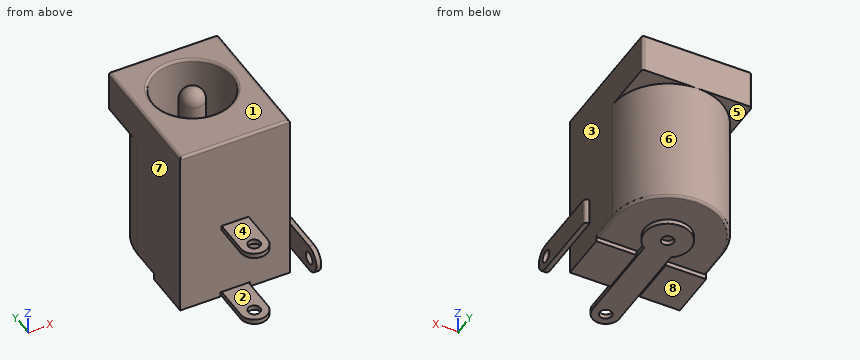
```python
from build123d import *

# Parameters (mm, degrees)
SKETCH1_W           = 9
SKETCH1_H           = 11
BOSS_EXTRUDE1_DEPTH = 3.3
BOSS_EXTRUDE2_DEPTH = 11
SKETCH3_R           = 3.25
CUT_EXTRUDE1_DEPTH  = 11
SKETCH4_R           = 1
BOSS_EXTRUDE3_DEPTH = 11
FILLET1_R           = 1
FILLET2_R           = 0.2
CUT_EXTRUDE2_DEPTH  = 0.4
SKETCH6_R           = 0.5
BOSS_EXTRUDE4_DEPTH = 0.4
SKETCH7_R           = 1.9
SKETCH7_R_2         = 0.5
BOSS_EXTRUDE5_DEPTH = 0.4
SKETCH8_R           = 0.5
BOSS_EXTRUDE6_DEPTH = 0.4
SKETCH9_R           = 0.5
BOSS_EXTRUDE7_DEPTH = 0.4
SKETCH10_W          = 2.8
SKETCH10_H          = 1
BOSS_EXTRUDE8_DEPTH = 6.4
FILLET3_R           = 0.3
FILLET4_R           = 0.2


with BuildPart() as part:
    # Sketch1 → Boss-Extrude1 (new body)
    with BuildSketch(Plane.XY):
        Rectangle(SKETCH1_W, SKETCH1_H)
    extrude(amount=-BOSS_EXTRUDE1_DEPTH)

    # Sketch2 → Boss-Extrude2 (add)
    with BuildSketch(Plane(origin=(0, 0, -3.3), x_dir=(-1, 0, 0), z_dir=(0, 0, -1))):
        with BuildLine():
            Line((-4.5, -5.5), (4.5, -5.5))
            Line((4.5, -5.5), (4.5, 1))
            ThreePointArc((4.5, 1), (0, 5.5), (-4.5, 1))
            Line((-4.5, 1), (-4.5, -5.5))
        make_face()
    extrude(amount=BOSS_EXTRUDE2_DEPTH)

    # Sketch3 → Cut-Extrude1 (cut)
    with BuildSketch(Plane.XY):
        with Locations((0, 1)):
            Circle(SKETCH3_R)
    extrude(amount=-CUT_EXTRUDE1_DEPTH, mode=Mode.SUBTRACT)

    # Sketch4 → Boss-Extrude3 (add)
    with BuildSketch(Plane.XY.offset(-11)):
        with Locations((0, 1)):
            Circle(SKETCH4_R)
    extrude(amount=BOSS_EXTRUDE3_DEPTH)

    # Fillet1
    fillet1_edges = [part.edges().sort_by_distance(p)[0] for p in [
        (-1, 1, 0),
    ]]
    fillet(fillet1_edges, radius=FILLET1_R)

    # Fillet2
    fillet2_edges = [part.edges().sort_by_distance(p)[0] for p in [
        (-3.25, 1, 0),
        (0, -5.5, 0),
        (-4.5, 0, 0),
        (0, 5.5, 0),
        (4.5, 0, 0),
        (-4.5, 5.5, -1.65),
        (4.5, 5.5, -1.65),
    ]]
    fillet(fillet2_edges, radius=FILLET2_R)

    # Sketch5 → Cut-Extrude2 (cut)
    with BuildSketch(Plane(origin=(0, 0, -14.3), x_dir=(-1, 0, 0), z_dir=(0, 0, -1))):
        Polygon((4.5, -1.5), (1.2, -1.5), (1.2, -5.5), (-1.2, -5.5), (-1.2, -1.5), (-4.5, -1.5), (-4.5, 5.5), (4.5, 5.5), align=None)
    extrude(amount=-CUT_EXTRUDE2_DEPTH, mode=Mode.SUBTRACT)

    # Sketch6 → Boss-Extrude4 (add)
    with BuildSketch(Plane(origin=(0, 0, -13.9), x_dir=(-1, 0, 0), z_dir=(0, 0, -1))):
        with BuildLine():
            Line((-1.1, -8.4), (-1.1, 1))
            ThreePointArc((-1.1, 1), (0, 2.1), (1.1, 1))
            Line((1.1, 1), (1.1, -8.4))
            ThreePointArc((1.1, -8.4), (0, -9.5), (-1.1, -8.4))
        make_face()
        with Locations((0, -8.4)):
            Circle(SKETCH6_R, mode=Mode.SUBTRACT)
        with Locations((0, 1)):
            Circle(SKETCH6_R, mode=Mode.SUBTRACT)
    extrude(amount=BOSS_EXTRUDE4_DEPTH)

    # Sketch7 → Boss-Extrude5 (add)
    with BuildSketch(Plane(origin=(0, 0, -14.3), x_dir=(-1, 0, 0), z_dir=(0, 0, -1))):
        with Locations((0, 1)):
            Circle(SKETCH7_R)
        with Locations((0, 1)):
            Circle(SKETCH7_R_2, mode=Mode.SUBTRACT)
    extrude(amount=-BOSS_EXTRUDE5_DEPTH)

    # Sketch8 → Boss-Extrude6 (add)
    with BuildSketch(Plane(origin=(0, 0, -8.1), x_dir=(-1, 0, 0), z_dir=(0, 0, -1))):
        with BuildLine():
            Line((-1.1, -5.145239298), (-1.1, -8.4))
            ThreePointArc((-1.1, -8.4), (0, -9.5), (1.1, -8.4))
            Line((1.1, -8.4), (1.1, -5.145239298))
            Line((1.1, -5.145239298), (-1.1, -5.145239298))
        make_face()
        with Locations((0, -8.4)):
            Circle(SKETCH8_R, mode=Mode.SUBTRACT)
    extrude(amount=-BOSS_EXTRUDE6_DEPTH)

    # Sketch9 → Boss-Extrude7 (add)
    with BuildSketch(Plane(origin=(4.5, 0, 0), x_dir=(0, 0, -1), z_dir=(1, 0, 0))):
        with BuildLine():
            Line((9.7, -2.5), (9.7, -8.4))
            ThreePointArc((9.7, -8.4), (10.8, -9.5), (11.9, -8.4))
            Line((11.9, -8.4), (11.9, -2.5))
            Line((11.9, -2.5), (9.7, -2.5))
        make_face()
        with Locations((10.8, -8.4)):
            Circle(SKETCH9_R, mode=Mode.SUBTRACT)
    extrude(amount=BOSS_EXTRUDE7_DEPTH)

    # Sketch10 → Boss-Extrude8 (add)
    with BuildSketch(Plane.XY.offset(-11)):
        with Locations((0, -2.25)):
            Rectangle(SKETCH10_W, SKETCH10_H)
    extrude(amount=BOSS_EXTRUDE8_DEPTH)

    # Fillet3
    fillet3_edges = [part.edges().sort_by_distance(p)[0] for p in [
        (4.9, -2.5, -10.8),
        (0, -1.75, -4.6),
    ]]
    fillet(fillet3_edges, radius=FILLET3_R)

    # Fillet4
    fillet4_edges = [part.edges().sort_by_distance(p)[0] for p in [
        (0, 5.5, -13.9),
        (4.5, -0.25, -13.9),
        (-4.5, -0.25, -13.9),
    ]]
    fillet(fillet4_edges, radius=FILLET4_R)


solid = part.part
```
Read the model definition and answer for the solid it produces. Units are mm, in the model's axes. Face numbers are marked on the shaded views. A direction names the side the tool comes from. Round coordinates to 2 decimals unless told otherwise and drop trailing zeros. Write each loop counter-clockwise with the first axis right and the second up, starting at its lowest first coordinate (ties: lowest second). Pieces come first, ordered by that corner, then holes. Notation, with made-up numbers: (4, 81) -> (13, 81) arc R24 ccw to (13, 117) -> close; hole circle Ø7 at (58, 14). An arc over 180 degrees is marked (long way). Answer in a Markdown table with one row per item. Add a question column.
1) Find section C-C, the plane z = -8.75. Determine the outline of the cut face in (x, y).
2) Given P1, Ø2.5, axis at x = 0, y = -8, coming from the +Z side; P2, Ø4, axis at x = -0.5, z = -8, coming from the -Y side; P3, Ø1.5, axis at y = -3, z = -6, coming from the +X side; P4, Ø0.7, axis at x = 3, z = -14, coming from the +Y side, each flat-ended and moving along its own axis, determine where each tip first touches the part or whether it passes through.
3) Determine the mould class of the marked faces 1, 2 and 3 for opening direction Z: pulls with the +Z half, pulls with the -Z half, needs draft (parallel to the pull), parting line crosses it, or undercut.
4) Find section A-A, the plane z = -1.75. Determine the outline of the cut face in (x, y).
5) Find section D-D, the plane z = -3.5. Determine the outline of the cut face in (x, y), and give its area (3 significant figures).
6) Which of the six approach directions +Z, -Z, +X, -X, +Y, -Y give full straight-line access (tool end or side, diameter ignored) to the marked faces 4, 5, 6, 7 and 8?
7) Consider line 1 (Y direction, x = 0, z = -14.05); line 2 (Y direction, x = 0, z = -7.9); line 3 (Y direction, x = 0, z = -5.75). Determine where each line is inside the solid, lowest interval first.
8) Find section B-B, the plane z = -10.8. Determine the outline of the cut face in (x, y).
Findings below:
| question | item | result |
|---|---|---|
| 1 | outline | (-4.5, -5.5) -> (4.5, -5.5) -> (4.5, 1) arc R4.5 ccw to (-4.5, 1) -> close; circle Ø2 at (0, 1); hole (-1.4, -1.93) -> (-1.4, -1.75) -> (1.4, -1.75) -> (1.4, -1.93) arc R3.25 ccw (long way) to start |
| 2 | P1 | z = -7.7 |
| 2 | P2 | y = -9.5 |
| 2 | P3 | x = 4.5 |
| 2 | P4 | y = 4.56 |
| 3 | face 1 | pulls with the +Z half |
| 3 | face 2 | undercut |
| 3 | face 3 | needs draft |
| 4 | outline | (-4.5, -5.5) -> (4.5, -5.5) -> (4.5, 5.3) arc R0.2 ccw to (4.3, 5.5) -> (-4.3, 5.5) arc R0.2 ccw to (-4.5, 5.3) -> close; circle Ø2 at (0, 1); hole circle Ø6.5 at (0, 1) |
| 5 | outline | (-4.5, -5.5) -> (4.5, -5.5) -> (4.5, 1) arc R4.5 ccw to (-4.5, 1) -> close; circle Ø2 at (0, 1); hole circle Ø6.5 at (0, 1) |
| 5 | area | 60.3 mm² |
| 6 | face 4 | +Z, +X, -X, -Y |
| 6 | face 5 | -Z, -X, +Y |
| 6 | face 6 | -Z, +Y |
| 6 | face 7 | +Z, -Z, -X, +Y, -Y |
| 6 | face 8 | -Z, +X, -X, +Y, -Y |
| 7 | line 1 | -9.5 to -8.9, -7.9 to 0.5, 1.5 to 2.9 |
| 7 | line 2 | -9.5 to -8.9, -7.9 to -1.75, 0 to 2, 4.25 to 5.5 |
| 7 | line 3 | -5.5 to -1.75, 0 to 2, 4.25 to 5.5 |
| 8 | outline | (-4.5, -5.5) -> (4.5, -5.5) -> (4.5, -7.9) -> (4.9, -7.9) -> (4.9, -2.8) arc R0.3 ccw to (4.6, -2.5) -> (4.5, -2.5) -> (4.5, 1) arc R4.5 ccw to (-4.5, 1) -> close; circle Ø2 at (0, 1); (4.5, -9.5) -> (4.9, -9.5) -> (4.9, -8.9) -> (4.5, -8.9) -> close; hole (-1.4, -1.93) -> (-1.4, -1.75) -> (1.4, -1.75) -> (1.4, -1.93) arc R3.25 ccw (long way) to start |
